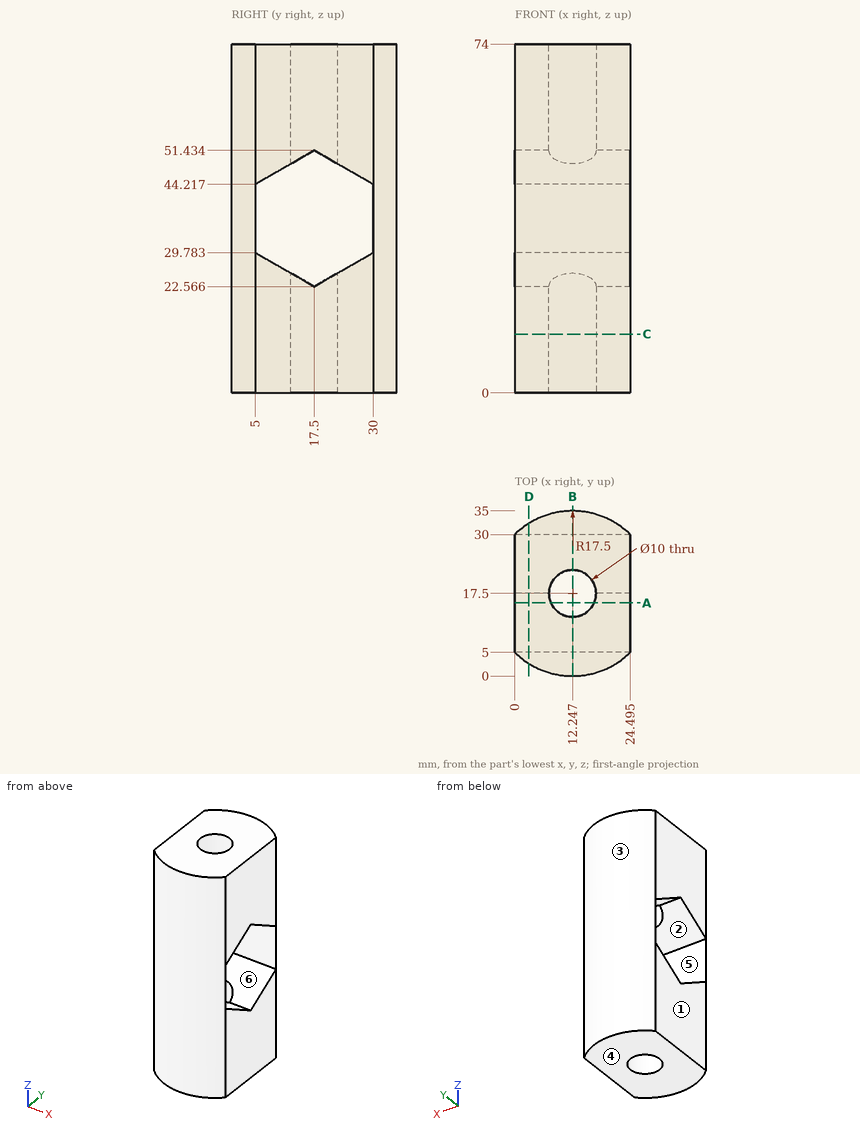
Print and shaded views of the part. All mm, measured from the part's lowest x, y and z. A direction names the side the tool comes from. Coordinates: 2 decimals unless noted, no trailing zeros. Order: outer loops, then holes, each group sorted by start corner. A loop starts at its lowest first (then second) coordinate and runs counter-clockwise, first axis right, second up. Notation, with made-up numbers: (82, 30.25) -> (113, 30.25) arc R25 ccw to (113, 65.25) -> close; hole circle Ø11 at (19, -19.5). An arc over 180 degrees is marked (long way). Answer as a JSON object with one key per item and string values. Group by question number.
1) Cut at C-C, the plane z = 12.5. Write the cut outline in (x, y) (1 decimal).
2) Flat gauge pins, fed straight in: pin 1 (6 mm diameter, centred on x = 12.25, y = 17.5, fed in from -Z); pin 2 (1.5 mm diameter, centred on x = 6, z = 53.5, fed in from +Y) (1 decimal); pin 3 (3 mm diameter, centred on x = 21.5, z = 62, fed in from +Y); pin 4 (10 mm diameter, centred on x = 18, z = 21, fed in from +Y). Where does each tip first touch, or does it go through?
3) Cut at B-B, the plane x = 12.25. Write the cut outline in (y, z).
4) Cut at A-A, the plane y = 15.5. Write the cut outline in (x, z) (1 decimal), then the cut area to 3 significant figures.
5) Cut at D-D, the plane x = 3. Write the cut outline in (y, z), then the cut area to 3 significant figures.
6) Drill centre lines: L1, parallel to X at y = 17.5, z = 7.5 (1 decimal); L2, parallel to X at y = 20, z = 9.5 (1 decimal); L3, parallel to Z at x = 17.75, y = 27. Where is each one in solid material? Low to high.
7) Which spindle directions (+Z, -Z, +X, -X, +Y, -Y) get a long thin tool onto all of the face, cutting with end or side? Do the marked faces 1 and 2. Say none if no direction does.
8) Pull direction Z, two halves, no side cores. Call the marked faces 3, 4, 5 and 6: +Z half, -Z half, draft (parallel to the pull), parting line (faces both ways), or undercut.
Check values:
{
 "1": {"outline": "(0, 5) arc R17.5 ccw to (24.5, 5) -> (24.5, 30) arc R17.5 ccw to (0, 30) -> close; hole circle Ø10 at (12.2, 17.5)"},
 "2": {"pin 1": "passes through", "pin 2": "stops at y = 34.1", "pin 3": "stops at y = 33.19", "pin 4": "stops at y = 34.98"},
 "3": {"outline": "(0, 0) -> (12.5, 0) -> (12.5, 25.45) -> (5, 29.78) -> (5, 44.22) -> (12.5, 48.55) -> (12.5, 74) -> (0, 74) -> close; (22.5, 0) -> (35, 0) -> (35, 74) -> (22.5, 74) -> (22.5, 48.55) -> (30, 44.22) -> (30, 29.78) -> (22.5, 25.45) -> close"},
 "4": {"outline": "(0, 0) -> (7.7, 0) -> (7.7, 23.7) -> (0, 23.7) -> close; (0, 50.3) -> (7.7, 50.3) -> (7.7, 74) -> (0, 74) -> close; (16.8, 0) -> (24.5, 0) -> (24.5, 23.7) -> (16.8, 23.7) -> close; (16.8, 50.3) -> (24.5, 50.3) -> (24.5, 74) -> (16.8, 74) -> close", "area": "727 mm²"},
 "5": {"outline": "(2.64, 0) -> (32.36, 0) -> (32.36, 74) -> (2.64, 74) -> close; hole (5, 29.78) -> (17.5, 22.57) -> (30, 29.78) -> (30, 44.22) -> (17.5, 51.43) -> (5, 44.22) -> close", "area": "1,660 mm²"},
 "6": {"L1": "x = 0 to 7.2, 17.2 to 24.5", "L2": "x = 0 to 7.9, 16.6 to 24.5", "L3": "z = 0 to 28.05, 45.95 to 74"},
 "7": {"face 1": "+Z, -Z, -X, +Y, -Y", "face 2": "+X, -X"},
 "8": {"face 3": "draft", "face 4": "-Z half", "face 5": "undercut", "face 6": "undercut"}
}
